```python
from build123d import *

# Parameters (mm, degrees)
F1_DEPTH = 76.2
F2_W     = 31.75
F2_H     = 25.4
F3_DEPTH = 6.35
F4_W     = 31.75
F4_H     = 25.4
F5_DEPTH = 6.35
F6_R     = 6.35
F7_DEPTH = 80.518


with BuildPart() as f1:
    # F0 (on Right) → F1 (new body)
    with BuildSketch(Plane.YZ):
        Polygon((0, 25.4), (0, 0), (50.8, 0), (88.9, 38.1), (88.9, 101.6), (63.5, 101.6), (63.5, 76.2), (44.45, 76.2), (18.9050504968, 50.8), (18.9050504968, 25.4), align=None)
    extrude(amount=F1_DEPTH)

    # F2 (on face) → F3 (cut)
    with BuildSketch(Plane.XZ.offset(-63.5)):
        with Locations((38.1, 88.9)):
            Rectangle(F2_W, F2_H)
    extrude(amount=-F3_DEPTH, mode=Mode.SUBTRACT)

    # F4 (on face) → F5 (cut)
    with BuildSketch(Plane.XZ):
        with Locations((38.735, 12.7)):
            Rectangle(F4_W, F4_H)
    extrude(amount=-F5_DEPTH, mode=Mode.SUBTRACT)

    # F6 (on face) → F7 (cut)
    with BuildSketch(Plane(origin=(0, -16.0008520758, 16.092163712), x_dir=(1, 0, 0), z_dir=(0, -0.7050920541, 0.7091157841))):
        with Locations((20.0781384668, 67.1823460538)):
            Circle(F6_R)
        with Locations((48.3754940052, 67.1823460538)):
            Circle(F6_R)
    extrude(amount=-F7_DEPTH, mode=Mode.SUBTRACT)


solid = f1.part
```
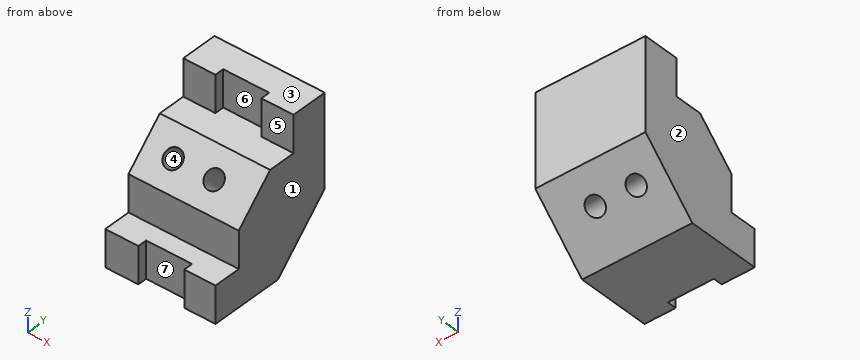
Geometry check sheet. Reference: the model listing, model coordinates, mm. Face numbers are marked on the shaded views. A direction names the side the tool comes from. Coordinates: 2 decimals unless noted, no trailing zeros. Order: outer loops, then holes, each group sorted by start corner. A loop starts at its lowest first (then second) coordinate and runs counter-clockwise, first axis right, second up. Notation, with made-up numbers: (42.25, -9) - (85.25, -9) arc R13 cw to (85.25, 11) - close; hole circle Ø2 at (-31, 64). An arc over 180 degrees is marked (long way). Answer as a JSON object with one key per item and string values. Group by question number.
Item 1: Depth check by flat-ended pin: pin 1 Ø5 at (y, z) = (3.5, 11) entering from -X; pin 2 Ø11 at (x, z) = (65.5, 90) entering from -Y; pin 3 Ø5.5 at (x, y) = (32.5, 13) entering from +Z; pin 4 Ø6 at (x, y) = (16, 79) entering from -Z. Enter the tip coordinate at first touch or a pass-through.
Item 2: Draft check along X on the marked faces 1, 2, 3 and 4. Enter one of: +X half, -X half, draft (parallel to the pull), parting line (faces both ways), or undercut.
Item 3: Sectioned sample at B-B, the plane z = 12. Record the cut outline in (x, y).
Item 4: Sectioned sample at C-C, the plane y = 81. Record the cut outline in (x, z).
Item 5: Tool access check on the marked faces 5, 6 and 7. Record the directions out of +Z, -Z, +X, -X, +Y, -Y that give a thin tool (end or side, any length) a straight path to the whole face; none if there is none.
Item 6: Sectioned sample at A-A, the plane x = 56.5. Record the cut outline in (y, z), and give its area (3 significant figures).
Item 7: Scan lines: probe 1 along X at (y, z) = (58, 45); probe 2 along Y at (x, z) = (31, 44); probe 3 along Y at (x, z) = (3, 86). Record each from-to range of solid material in increasing order.
Item 8: Sectioned sample at D-D, the plane y = 66.5. Give the number of separate pieces and of enclosed holes in the cut face, and give its area (3 significant figures).
Resolved:
{
 "1": {"pin 1": "x = 0", "pin 2": "y = 63.5", "pin 3": "z = 25.4", "pin 4": "z = 25.23"},
 "2": {"face 1": "+X half", "face 2": "-X half", "face 3": "draft", "face 4": "undercut"},
 "3": {"outline": "(0, 0) - (22.86, 0) - (22.86, 6.35) - (54.61, 6.35) - (54.61, 0) - (76.2, 0) - (76.2, 62.8) - (0, 62.8) - close"},
 "4": {"outline": "(0, 30.2) - (76.2, 30.2) - (76.2, 101.6) - (0, 101.6) - close"},
 "5": {"face 5": "+Z, +X, -X, -Y", "face 6": "+Z, -Y", "face 7": "+Z, -Z, -Y"},
 "6": {"outline": "(0, 0) - (50.8, 0) - (88.9, 38.1) - (88.9, 101.6) - (63.5, 101.6) - (63.5, 76.2) - (44.45, 76.2) - (18.91, 50.8) - (18.91, 25.4) - (0, 25.4) - close", "area": "5,410 mm^2"},
 "7": {"probe 1": "0 to 17.23, 22.93 to 45.53, 51.22 to 76.2", "probe 2": "18.91 to 88.9", "probe 3": "63.5 to 88.9"},
 "8": {"separate pieces": "1", "enclosed holes": "2", "area": "5,380 mm^2"}
}
